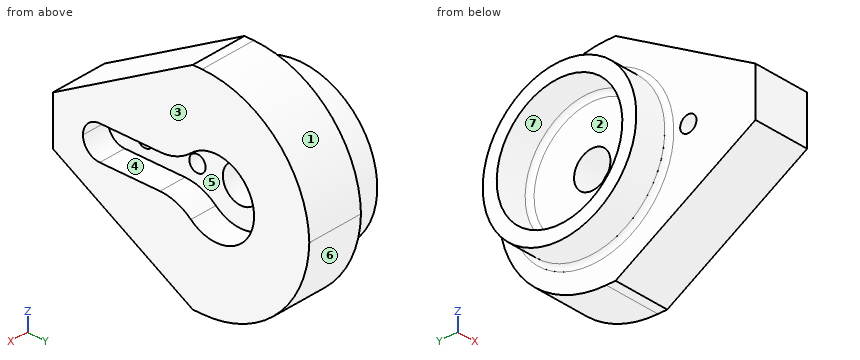
from build123d import *

# Parameters (mm, degrees)
SKETCH1_W           = 20
SKETCH1_H           = 20
BOSS_EXTRUDE1_DEPTH = 20
SKETCH2_W           = 45
SKETCH2_H           = 70
BOSS_EXTRUDE2_DEPTH = 12
CUT_EXTRUDE1_DEPTH  = 5.8
FILLET1_R           = 3.6
FILLET2_R           = 10
SKETCH5_R           = 3.9
CUT_EXTRUDE2_DEPTH  = 53.490475326
CUT_EXTRUDE3_REACH  = 51.17
SKETCH6_R           = 1.75
SKETCH13_W          = 20
SKETCH13_H          = 20
CUT_EXTRUDE9_DEPTH  = 20
SKETCH14_R          = 16.475
BOSS_EXTRUDE3_DEPTH = 7.6
SKETCH15_W          = 12
SKETCH15_H          = 45
CUT_EXTRUDE10_DEPTH = 15
FILLET3_R           = 23
CHAMFER1_SIZE       = 30
CHAMFER1_SIZE2      = 17.320508076
CHAMFER2_SIZE       = 30
CHAMFER2_SIZE2      = 17.320508076
SKETCH16_R          = 13.475
CUT_EXTRUDE11_DEPTH = 7.6
FILLET4_R           = 1


# Some blends are built 0.0001 mm under size
with BuildPart() as part:
    # Sketch1 → Boss-Extrude1 (new body)
    with BuildSketch(Plane(origin=(0, 0, 0), x_dir=(0, 0, -1), z_dir=(1, 0, 0))):
        Rectangle(SKETCH1_W, SKETCH1_H)
    extrude(amount=BOSS_EXTRUDE1_DEPTH)

    # Sketch2 → Boss-Extrude2 (add)
    with BuildSketch(Plane(origin=(20, 0, 0), x_dir=(0, 0, -1), z_dir=(1, 0, 0))):
        Rectangle(SKETCH2_W, SKETCH2_H)
    extrude(amount=BOSS_EXTRUDE2_DEPTH)

    # Sketch4 → Cut-Extrude1 (cut)
    with BuildSketch(Plane(origin=(32, 0, 0), x_dir=(0, 0, -1), z_dir=(1, 0, 0))):
        with BuildLine():
            Line((3.6, -28.55), (-3.6, -28.55))
            Line((-3.6, -28.55), (-3.6, -7.311805523))
            ThreePointArc((-3.6, -7.311805523), (0, 8.15), (3.6, -7.311805523))
            Line((3.6, -7.311805523), (3.6, -28.55))
        make_face()
    extrude(amount=-CUT_EXTRUDE1_DEPTH, mode=Mode.SUBTRACT)

    # Fillet1
    fillet1_edges = [part.edges().sort_by_distance(p)[0] for p in [
        (29.1, -28.55, 3.6),
        (29.1, -28.55, -3.6),
    ]]
    fillet(fillet1_edges, radius=FILLET1_R - 0.0001)  # a hair under: the kernel refuses the full size

    # Fillet2
    fillet2_edges = [part.edges().sort_by_distance(p)[0] for p in [
        (29.1, -7.311805523, 3.6),
        (29.1, -7.311805523, -3.6),
    ]]
    fillet(fillet2_edges, radius=FILLET2_R)

    # Sketch5 → Cut-Extrude2 (cut, through all)
    with BuildSketch(Plane.ZY):
        Circle(SKETCH5_R)
    extrude(amount=-CUT_EXTRUDE2_DEPTH, mode=Mode.SUBTRACT)

    # Sketch6 → Cut-Extrude3 (cut, up to next)
    with BuildSketch(Plane(origin=(26.2, 0, 0), x_dir=(0, 0, -1), z_dir=(1, 0, 0)), mode=Mode.PRIVATE) as cut_extrude3_sk1:
        with Locations((0, -20.6)):
            Circle(SKETCH6_R)
    cut_extrude3_tool1 = extrude(cut_extrude3_sk1.sketch, amount=-CUT_EXTRUDE3_REACH, mode=Mode.PRIVATE) & part.part
    # Sketch6 → Cut-Extrude3 (cut, up to next)
    with BuildSketch(Plane(origin=(26.2, 0, 0), x_dir=(0, 0, -1), z_dir=(1, 0, 0)), mode=Mode.PRIVATE) as cut_extrude3_sk2:
        with Locations((0, -9.35)):
            Circle(SKETCH6_R)
    cut_extrude3_tool2 = extrude(cut_extrude3_sk2.sketch, amount=-CUT_EXTRUDE3_REACH, mode=Mode.PRIVATE) & part.part
    add(cut_extrude3_tool1.solids().sort_by_distance((26.2, -20.6, 0))[0], mode=Mode.SUBTRACT)
    add(cut_extrude3_tool2.solids().sort_by_distance((26.2, -9.35, 0))[0], mode=Mode.SUBTRACT)

    # Sketch13 → Cut-Extrude9 (cut)
    with BuildSketch(Plane.ZY):
        Rectangle(SKETCH13_W, SKETCH13_H)
    extrude(amount=-CUT_EXTRUDE9_DEPTH, mode=Mode.SUBTRACT)

    # Sketch14 → Boss-Extrude3 (add)
    with BuildSketch(Plane.ZY.offset(-20)):
        with Locations(Location((0, 0, 0), (0, 0, 180))):
            Circle(SKETCH14_R)
    extrude(amount=BOSS_EXTRUDE3_DEPTH)

    # Sketch15 → Cut-Extrude10 (cut)
    with BuildSketch(Plane(origin=(0, 35, 0), x_dir=(1, 0, 0), z_dir=(0, 1, 0))):
        with Locations((26, 0)):
            Rectangle(SKETCH15_W, SKETCH15_H)
    extrude(amount=-CUT_EXTRUDE10_DEPTH, mode=Mode.SUBTRACT)

    # Fillet3
    # the kernel refuses this fillet: 23 mm, written as the material it takes off along each edge
    with BuildSketch(Plane(origin=(-37.5, 20, -22.5), x_dir=(0, -1, 0), z_dir=(1, 0, 0)), Plane(origin=(89.5, 20, 22.5), x_dir=(0, -1, 0), z_dir=(-1, 0, 0))) as fillet3_piece_1:
        with BuildLine():
            CenterArc((FILLET3_R, -FILLET3_R), FILLET3_R, 90, 90)
            Line((0, -FILLET3_R), (0, 0))
            Line((0, 0), (FILLET3_R, 0))
        make_face()
    extrude(amount=127, mode=Mode.SUBTRACT)

    # Chamfer1
    chamfer1_edges = [part.edges().sort_by_distance(p)[0] for p in [
        (26, -35, 22.5),
    ]]
    chamfer1_side = [part.faces().sort_by_distance(p)[0] for p in [
        (26, -19, 22.5),
    ]]
    chamfer(chamfer1_edges, length=CHAMFER1_SIZE, length2=CHAMFER1_SIZE2, reference=chamfer1_side[0])

    # Chamfer2
    chamfer2_edges = [part.edges().sort_by_distance(p)[0] for p in [
        (26, -35, -22.5),
    ]]
    chamfer2_side = [part.faces().sort_by_distance(p)[0] for p in [
        (26, -19, -22.5),
    ]]
    chamfer(chamfer2_edges, length=CHAMFER2_SIZE, length2=CHAMFER2_SIZE2, reference=chamfer2_side[0])

    # Sketch16 → Cut-Extrude11 (cut)
    with BuildSketch(Plane.ZY.offset(-12.4)):
        Circle(SKETCH16_R)
    extrude(amount=-CUT_EXTRUDE11_DEPTH, mode=Mode.SUBTRACT)

    # Fillet4
    fillet4_edges = [part.edges().sort_by_distance(p)[0] for p in [
        (20, 0, 16.475),
        (20, 0, -13.475),
    ]]
    fillet(fillet4_edges, radius=FILLET4_R)


solid = part.part
Verification items for the finished model (mm, model axes). Face numbers are marked on the shaded views. A direction names the side the tool comes from. Coordinates: 2 decimals unless noted, no trailing zeros. Order: outer loops, then holes, each group sorted by start corner. A loop starts at its lowest first (then second) coordinate and runs counter-clockwise, first axis right, second up. Notation, with made-up numbers: (89.5, 77) -> (112.5, 77) arc R26 ccw to (112.5, 112) -> close; hole circle Ø9 at (57, 23.25). An arc over 180 degrees is marked (long way). Put each result on its own line as item: value. Start each with the question number.
1. Material ranges on L1, parallel to Y at x = 26, z = 1; L2, parallel to Y at x = 29.75, z = -1; L3, parallel to Z at x = 27.85, y = 0, recorded low to high. Write a range as [from, to].
2. Cross-section at D-D, the plane z = 19.5. Record the boundary of the cut face in (x, y), then the cut area to 3 significant figures.
3. Cross-section at C-C, the plane x = 17.5. Record the boundary of the cut face in (y, z) (3 decimals).
4. Cross-section at B-B, the plane x = 21.25. Record the boundary of the cut face in (y, z), then the cut area to 3 significant figures.
5. Mould release check, pull along Z, two halves, no side actions. Record for the marked faces 1, 2, 3 and 4: released by +Z, released by -Z, zero draft, split by the parting line, or undercut.
6. Go/stop test with flat-tipped pins: pin 1 Ø5 at (y, z) = (-8, 0) entering from +X; pin 2 Ø1 at (y, z) = (4, -10.5) entering from -X; pin 3 Ø6 at (x, y) = (25, 7) entering from +Z. Record where each tip stops, or that it passes through.
7. Access from +Z, -Z, +X, -X, +Y, -Y to the whole of each face (thin tool, end or side, straight path). Record for the marked faces 5, 6 and 7.
Computed:
1. L1: [-35, -22.04], [-19.16, -10.79], [-7.91, -3.77], [3.77, 19.95]
1. L2: [-35, -28.41], [8.09, 19.95]
1. L3: [-22.3, -8.15], [8.15, 22.3]
2. outline: (20, -10.2) -> (32, -10.2) -> (32, 8.36) -> (20, 8.36) -> close
2. area: 223 mm2
3. outline: circle Ø32.95 at (0, 0); hole circle Ø26.95 at (0, 0)
4. outline: (-35, -5.18) -> (-5, -22.5) -> (-3, -22.5) arc R23 ccw to (19.99, 0) arc R23 ccw to (-3, 22.5) -> (-5, 22.5) -> (-35, 5.18) -> close; hole circle Ø3.5 at (-20.6, 0); hole circle Ø3.5 at (-9.35, 0); hole circle Ø7.8 at (0, 0)
4. area: 1,660 mm2
5. face 1: released by +Z
5. face 2: undercut
5. face 3: zero draft
5. face 4: undercut
6. pin 1: x = 26.2
6. pin 2: x = 20
6. pin 3: z = 21.41
7. face 5: +X
7. face 6: -Z, +X, -X, +Y
7. face 7: -X
